Here's the drawing with two shaded views (mm, measured from the low corner). I have some questions. A direction names the side the tool comes from. Coordinates: 2 decimals unless noted, no trailing zeros. Loops run counter-clockwise (first coordinate to the right, second up) from the corner with the lowest first, then second, coordinate; pieces in that order, holes last. Notation, with made-up numbers: M 9,59 L 41,59 A9 cw 41,70 Z; hole C 65.5,-23.75 d8. An arc over 180 degrees is marked long. Use one line per item in the form item = value. Start each with the question number.
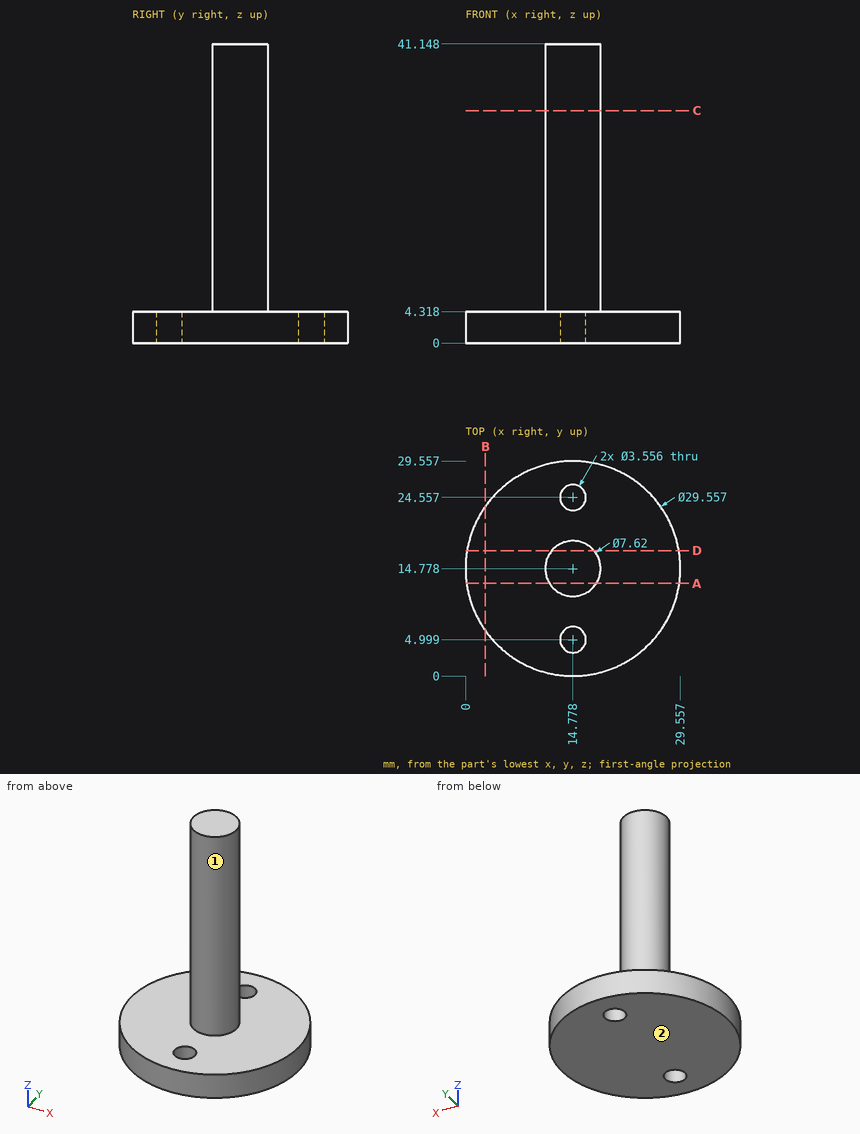
Item 1: I want a section at B-B (x = 2.75). Write out the boundary of the cut face in (y, z) (1 decimal).
Item 2: For the marked faces 1 and 2, which set-ups out of +Z, -Z, +X, -X, +Y, -Y let a thin tool reach every point of the face, with its end or its side?
Item 3: I want a section at C-C (z = 32). Write out the boundary of the cut face in (x, y), plus the area to 3 significant figures.
Item 4: I want a section at A-A (y = 12.75). Write out the boundary of the cut face in (x, z).
Item 5: Please list where these lines run through material, in increasing order: line 1 along Z through (x, y) = (11.5, 22.25); line 2 along X through (y, z) = (24.75, 3) (1 decimal); line 3 along X through (y, z) = (14.5, 32).
Item 6: I'm going to push flat-ended pins straight in: P1, Ø2, axis at y = 8, z = 26.5, coming from the -X side; P2, Ø1, axis at x = 25.5, y = 10.5, coming from the -Z side; P3, Ø4, axis at y = 12, z = 36.5, coming from the -X side. Where does each tip first touch, or does it pass through?
Item 7: I want a section at D-D (y = 17.25). Write out the boundary of the cut face in (x, z).
Worked answers:
q1.outline = M 6.2,0 L 23.4,0 L 23.4,4.3 L 6.2,4.3 Z
q2.face_1 = +Z
q2.face_2 = -Z, +X, -X, +Y, -Y
q3.outline = C 14.78,14.78 d7.62
q3.area = 45.6 mm²
q4.outline = M 0.14,0 L 29.42,0 L 29.42,4.32 L 18,4.32 L 18,41.15 L 11.55,41.15 L 11.55,4.32 L 0.14,4.32 Z
q5.line_1 = 0 to 4.32
q5.line_2 = 3.9 to 13, 16.5 to 25.7
q5.line_3 = 10.98 to 18.58
q6.P1 = through
q6.P2 = 0
q6.P3 = 11.05
q7.outline = M 0.21,0 L 29.35,0 L 29.35,4.32 L 17.68,4.32 L 17.68,41.15 L 11.88,41.15 L 11.88,4.32 L 0.21,4.32 Z
